```python
from build123d import *

# Parameters (mm, degrees)
F0_W     = 127
F0_H     = 127
F1_DEPTH = 19.05
F3_DEPTH = 2.54


with BuildPart() as f1:
    # F0 (on Top) → F1 (new body)
    with BuildSketch(Plane.XY):
        Rectangle(F0_W, F0_H)
    extrude(amount=F1_DEPTH)

    # F2 (on face) → F3 (cut)
    with BuildSketch(Plane.XY.offset(19.05)):
        Polygon((6.411221, -17.744777), (6.411221, 17.744777), (-10.465065, 23.228214), (-15.868622, 24.983937), (-20.305928, 26.425704), (-27.34135, 28.711652), (-48.201586, 0), (-27.34135, -28.711652), align=None)
        with BuildLine():
            Line((-10.465065, 23.228214), (6.411221, 17.744777))
            ThreePointArc((6.411221, 17.744777), (-5.946353, 25.166002), (-20.305928, 26.425704))
            Line((-20.305928, 26.425704), (-15.868622, 24.983937))
            ThreePointArc((-15.868622, 24.983937), (-13.055853, 24.44767), (-10.465065, 23.228214))
        make_face()
    extrude(amount=-F3_DEPTH, mode=Mode.SUBTRACT)


solid = f1.part
```
Here's how the part is built. I have some questions about the finished solid (model axes, mm). A direction names the side the tool comes from. Coordinates: 2 decimals unless noted, no trailing zeros. Order: outer loops, then holes, each group sorted by start corner. A loop starts at its lowest first (then second) coordinate and runs counter-clockwise, first axis right, second up.
Item 1: Thinking about a two-plate mould opening in Y: for faces 3 (the face through (63.5, -1, 9)), 4 (the face through (-10.701, -23.305, 17.798)), 5 (the face through (-1, -63.5, 9)), which applies, pulls with the +Y half, pulls with the -Y half, needs draft (parallel to the pull), parting line crosses it, or undercut?
Response values:
face 3: needs draft
face 4: undercut
face 5: pulls with the -Y half
Item 2: If we section it at C-C, the plane x = -12.5: List the corners of the cut face in (y, z) for me.
Response values:
outline: (-63.5, 0) - (63.5, 0) - (63.5, 19.05) - (26.56, 19.05) - (26.56, 16.51) - (24.25, 16.51) - (24.25, 19.05) - (23.89, 19.05) - (23.89, 16.51) - (-23.89, 16.51) - (-23.89, 19.05) - (-63.5, 19.05) - close
Item 3: Which directions (+Z, -Z, +X, -X, +Y, -Y) give clear straight access to the entire face, cutting with the end or side of a thin tool? Please do faces 1 (the face through (-5.75, 25.1, 17.8)), 2 (the face through (-1, 1, 0)).
Response values:
face 1: +Z
face 2: -Z, +X, -X, +Y, -Y
Item 4: I'm going to push a flat-ended pin straight in: pin 1 Ø3 at (x, y) = (-28, 22.5) entering from +Z. Where does the tip first touch, or does it pass through?
Response values:
pin 1: stops at z = 16.51
Item 5: I need wall thicknesses on probe 1 along X at (y, z) = (20.5, 17.25); probe 2 along X at (y, z) = (16.5, 17.25); probe 3 along Y at (x, z) = (-41, 17.5). Which ranges of each line are inside material? Lowest first, please.
Response values:
probe 1: x = -63.5 to -33.31, 3.15 to 63.5
probe 2: x = -63.5 to -36.21, 6.41 to 63.5
probe 3: y = -63.5 to -9.91, 9.91 to 63.5
Item 6: If we section it at B-B, the plane y = 7.5: List the corners of the cut face in (x, z) for me.
Response values:
outline: (-63.5, 0) - (63.5, 0) - (63.5, 19.05) - (6.41, 19.05) - (6.41, 16.51) - (-42.75, 16.51) - (-42.75, 19.05) - (-63.5, 19.05) - close
Item 7: If we section it at A-A, the plane x = 4: List the corners of the cut face in (y, z) for me.
Response values:
outline: (-63.5, 0) - (63.5, 0) - (63.5, 19.05) - (19.85, 19.05) - (19.85, 16.51) - (-18.53, 16.51) - (-18.53, 19.05) - (-63.5, 19.05) - close
